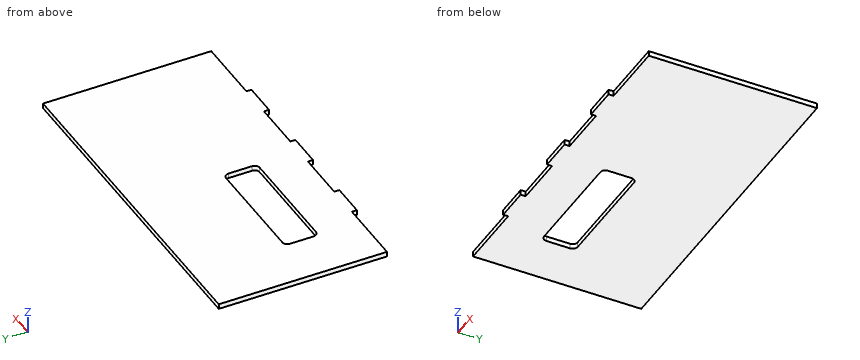
from build123d import *

# Parameters (mm, degrees)
BOSS_EXTRUDE1_DEPTH = 3


with BuildPart() as part:
    # Sketch1 → Boss-Extrude1 (new body)
    with BuildSketch(Plane.XY):
        Polygon((-100, -50), (-60, -50), (-60, -53), (-40, -53), (-40, -50), (-10, -50), (-10, -53), (10, -53), (10, -50), (40, -50), (40, -53), (60, -53), (60, -50), (100, -50), (100, 50), (-100, 50), align=None)
        with BuildLine():
            Line((-67, -25), (-3, -25))
            ThreePointArc((-3, -25), (-0.878679656, -24.121320344), (0, -22))
            Line((0, -22), (0, -8))
            ThreePointArc((0, -8), (-0.878679656, -5.878679656), (-3, -5))
            Line((-3, -5), (-67, -5))
            ThreePointArc((-67, -5), (-69.121320344, -5.878679656), (-70, -8))
            Line((-70, -8), (-70, -22))
            ThreePointArc((-70, -22), (-69.121320344, -24.121320344), (-67, -25))
        make_face(mode=Mode.SUBTRACT)
    extrude(amount=BOSS_EXTRUDE1_DEPTH)


solid = part.part
The listing builds one solid part. Answer for the finished solid, in the listing's coordinates (mm). Round coordinates to 2 decimals unless told otherwise and drop trailing zeros. Loops run counter-clockwise (first coordinate to the right, second up) from the corner with the lowest first, then second, coordinate; pieces in that order, holes last. Notation, with made-up numbers: M -2.75,-26 L 48.25,-26 A19 ccw 48.25,10 Z; hole C 85,26 d1. An arc over 180 degrees is marked long. Write each question's results on one line, items separated by ' | '. Start each with the question number.
1) Straight lines are drawn through the part: probe 1 along X at (y, z) = (-19, 1.05); probe 2 along Y at (x, z) = (-21, 1.9); probe 3 along Y at (x, z) = (61, 0.95). For each, find the intervals that lie inside material, in ascending order.
2) Find section B-B on z = 1. Write down the section's boundary in (x, y), plus the area to 3 significant figures.
3) Find section C-C on x = 16. Write down the section's boundary in (y, z), plus the area to 3 significant figures.
4) Find section A-A on x = -7.5. Write down the section's boundary in (y, z).
5) Each of these flat-tipped pins is pushed along its axis until it touches: pin 1 (1.5 mm diameter, centred on y = -51, z = 1, fed in from +X); pin 2 (0.9 mm diameter, centred on x = 26.5, z = 2, fed in from -Y). Where does it stop, or does it pass through?
Final values:
1) probe 1: -100 to -70, 0 to 100 | probe 2: -50 to -25, -5 to 50 | probe 3: -50 to 50
2) outline: M -100,-50 L -60,-50 L -60,-53 L -40,-53 L -40,-50 L -10,-50 L -10,-53 L 10,-53 L 10,-50 L 40,-50 L 40,-53 L 60,-53 L 60,-50 L 100,-50 L 100,50 L -100,50 Z; hole M -70,-22 A3 ccw -67,-25 L -3,-25 A3 ccw 0,-22 L 0,-8 A3 ccw -3,-5 L -67,-5 A3 ccw -70,-8 Z | area: 18,800 mm²
3) outline: M -50,0 L 50,0 L 50,3 L -50,3 Z | area: 300 mm²
4) outline: M -53,0 L -25,0 L -25,3 L -53,3 Z; M -5,0 L 50,0 L 50,3 L -5,3 Z
5) pin 1: x = 60 | pin 2: y = -50
